Job drawing, mm, ordinate dimensions from the low corner. One solid piece. Round coordinates to 2 decimals unless told otherwise and drop trailing zeros. Write each loop counter-clockwise with the first axis right and the second up, starting at its lowest first coordinate (ties: lowest second). Pieces come first, ordered by that corner, then holes. Notation, with made-up numbers: (84, -4) -> (95, -4) arc R19 cw to (95, 13) -> close; hole circle Ø8 at (37, 16.5). An arc over 180 degrees is marked (long way). Use CSV: the item, a comma, the result in double quotes. Start each with the question number.
(1) Saw through at D-D (y = 46.5). Give the cut face in (x, z), plus the area to 3 significant figures.
(2) Saw through at A-A (x = 114.3). Count the separate pieces of the cut face and the enclosed holes in it.
(3) Probe line 1 (Z direction, x = 114, y = 296) (1 decimal); line 2 (X direction, y = 93, z = 114.3); line 3 (Y direction, x = 96, z = 19). List the from-to ranges inside material, lowest first. Write a range as [from, to].
(4) Saw through at B-B (z = 114.3). Give the cut face in (x, y), plus the area to 3 significant figures.
(5) Drop flat-ended pins along their axis: pin 1 (1.5 mm diameter, centred on x = 173, y = 131.5, fed in from +Z); pin 2 (2 mm diameter, centred on y = 270, z = 160.5, fed in from -X); pin 3 (4 mm diameter, centred on x = 167.5, y = 242, fed in from +Z); pin 4 (6 mm diameter, centred on x = 129, z = 184, fed in from +Y). Give the stop position or say it passes through.
(6) Two-plate mould, pull along Y, no slides. Class the marked faces 1, 2, 3 and 4: released by +Y, released by -Y, zero draft, split by the parting line, or undercut.
(7) Saw through at C-C (x = 20.5). Give the cut face in (y, z) (3 decimals), plus the area to 3 significant figures.
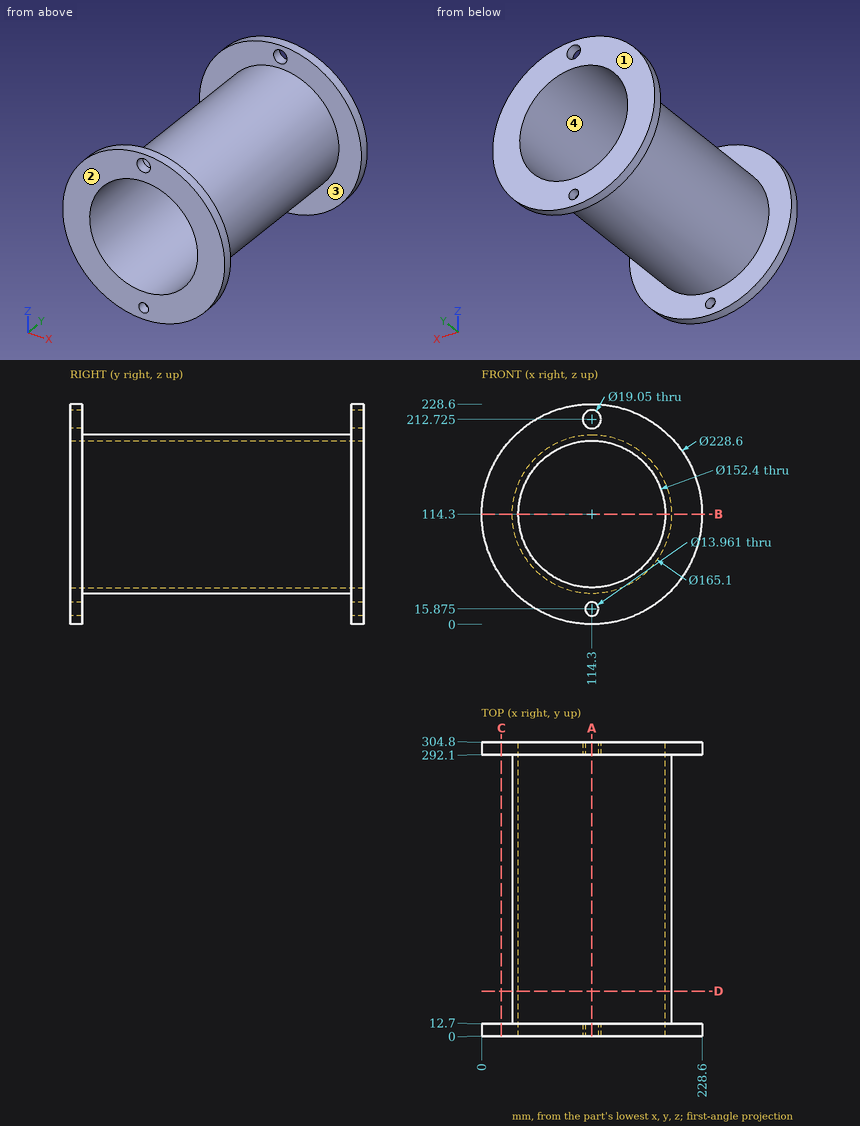
Answers:
1,outline,"circle Ø165.1 at (114.3, 114.3); hole circle Ø152.4 at (114.3, 114.3)"
1,area,"3,170 mm²"
2,separate pieces,"6"
2,enclosed holes,"0"
3,line 1,"z = [0, 8.9], [22.8, 38.1], [190.5, 203.2], [222.2, 228.6]"
3,line 2,"x = [31.75, 38.1], [190.5, 196.85]"
3,line 3,"y = [0, 12.7], [292.1, 304.8]"
4,outline,"(0, 0) -> (38.1, 0) -> (38.1, 304.8) -> (0, 304.8) -> (0, 292.1) -> (31.75, 292.1) -> (31.75, 12.7) -> (0, 12.7) -> close; (190.5, 0) -> (228.6, 0) -> (228.6, 12.7) -> (196.85, 12.7) -> (196.85, 292.1) -> (228.6, 292.1) -> (228.6, 304.8) -> (190.5, 304.8) -> close"
4,area,"5,480 mm²"
5,pin 1,"stops at z = 173.09"
5,pin 2,"stops at x = 45.22"
5,pin 3,"stops at z = 179.05"
5,pin 4,"passes through"
6,face 1,"released by +Y"
6,face 2,"released by -Y"
6,face 3,"undercut"
6,face 4,"zero draft"
7,outline,"(0, 48.985) -> (12.7, 48.985) -> (12.7, 179.615) -> (0, 179.615) -> close; (292.1, 48.985) -> (304.8, 48.985) -> (304.8, 179.615) -> (292.1, 179.615) -> close"
7,area,"3,320 mm²"
